```python
from build123d import *

# Parameters (mm, degrees)
SKETCH1_R               = 12
BOSS_EXTRUDE1_DEPTH     = 12
SKETCH9_R               = 14.1
CUT_EXTRUDE2_DEPTH      = 9
SKETCH7_R               = 14
SKETCH7_R_2             = 12
BOSS_EXTRUDE3_DEPTH     = 3
CUT_EXTRUDE5_DEPTH      = 49.191389272
CUT_EXTRUDE5_DEPTH_BACK = 49.191389272
SKETCH12_R              = 1.6
SKETCH13_W              = 2.5
SKETCH13_H              = 1
CUT_EXTRUDE6_DEPTH      = 9
CHAMFER1_SIZE           = 0.6
CHAMFER1_SIZE_2         = 0.661222502


with BuildPart() as part:
    # Sketch1 → Boss-Extrude1 (new body)
    with BuildSketch(Plane.XY):
        with BuildLine():
            Line((-15.1, -38), (-10.1, -38))
            Line((-10.1, -38), (-10.1, -20))
            Line((-10.1, -20), (10.1, -20))
            Line((10.1, -20), (10.1, -38))
            Line((10.1, -38), (15.1, -38))
            Line((15.1, -38), (15.1, -11.029534738))
            ThreePointArc((15.1, -11.029534738), (15.331712472, -8.319532432), (16.020123134, -5.688203124))
            ThreePointArc((16.020123134, -5.688203124), (0, 17), (-16.020123134, -5.688203124))
            ThreePointArc((-16.020123134, -5.688203124), (-15.331712472, -8.319532432), (-15.1, -11.029534738))
            Line((-15.1, -11.029534738), (-15.1, -38))
        make_face()
        Circle(SKETCH1_R, mode=Mode.SUBTRACT)
    extrude(amount=BOSS_EXTRUDE1_DEPTH)

    # Sketch9 → Cut-Extrude2 (cut)
    with BuildSketch(Plane.XY.offset(12)):
        Circle(SKETCH9_R)
    extrude(amount=-CUT_EXTRUDE2_DEPTH, mode=Mode.SUBTRACT)

    # Sketch7 → Boss-Extrude3 (add)
    with BuildSketch(Plane.XY):
        Circle(SKETCH7_R)
        with Locations(Location((0, 0, 0), (0, 0, 180))):
            Circle(SKETCH7_R_2, mode=Mode.SUBTRACT)
    extrude(amount=BOSS_EXTRUDE3_DEPTH)

    # Sketch12 → Cut-Extrude5 (cut, two sides: drawn at the far end of the back side and taken through both)
    with BuildSketch(Plane.ZY.offset(-10.1).offset(-CUT_EXTRUDE5_DEPTH_BACK)):
        with Locations(Location((6, -30, 0), (0, 0, 270))):
            Circle(SKETCH12_R)
    extrude(amount=CUT_EXTRUDE5_DEPTH + CUT_EXTRUDE5_DEPTH_BACK, mode=Mode.SUBTRACT)

    # Sketch13 → Cut-Extrude6 (cut)
    with BuildSketch(Plane.XY.offset(12)):
        with Locations((0, -14.544482903)):
            Rectangle(SKETCH13_W, SKETCH13_H)
    extrude(amount=-CUT_EXTRUDE6_DEPTH, mode=Mode.SUBTRACT)

    # Chamfer1
    # the kernel refuses this chamfer: 0.661222502, 0.6 mm, written as the material it takes off along each edge
    with BuildSketch(Plane(origin=(10.1, -20, 0), x_dir=(0, 0, 1), z_dir=(0, -1, 0)), Plane(origin=(-10.1, -39.543009793, 0), x_dir=(0, 0, 1), z_dir=(0, 1, 0))) as chamfer1_piece_1:
        Polygon((CHAMFER1_SIZE, 0), (0, -CHAMFER1_SIZE), (0, 0), align=None)
    extrude(amount=19.543009793, mode=Mode.SUBTRACT)
    with BuildSketch(Plane(origin=(-10.1, -20, 0), x_dir=(0, 0, 1), z_dir=(1, 0, 0))) as chamfer1_piece_2:
        Polygon((CHAMFER1_SIZE, 0), (0, -CHAMFER1_SIZE), (0, 0), align=None)
    extrude(amount=20.2, mode=Mode.SUBTRACT)
    with BuildSketch(Plane(origin=(-10.1, -39.543009793, 12), x_dir=(0, 0, -1), z_dir=(0, 1, 0)), Plane(origin=(10.1, -20, 12), x_dir=(0, 0, -1), z_dir=(0, -1, 0))) as chamfer1_piece_3:
        Polygon((CHAMFER1_SIZE, 0), (0, CHAMFER1_SIZE), (0, 0), align=None)
    extrude(amount=19.543009793, mode=Mode.SUBTRACT)
    with BuildSketch(Plane(origin=(10.1, -38, -1.543009793), x_dir=(0, 1, 0), z_dir=(0, 0, 1))) as chamfer1_piece_4:
        Polygon((CHAMFER1_SIZE, 0), (0, -CHAMFER1_SIZE), (0, 0), align=None)
    extrude(amount=15.086019586, mode=Mode.SUBTRACT)
    with BuildSketch(Plane(origin=(-10.1, -38, -1.543009793), x_dir=(0, 1, 0), z_dir=(0, 0, 1))) as chamfer1_piece_5:
        Polygon((CHAMFER1_SIZE, 0), (0, CHAMFER1_SIZE), (0, 0), align=None)
    extrude(amount=15.086019586, mode=Mode.SUBTRACT)
    with BuildSketch(Plane(origin=(-10.1, -20, 12), x_dir=(0, 0, -1), z_dir=(1, 0, 0))) as chamfer1_piece_6:
        Polygon((CHAMFER1_SIZE, 0), (0, CHAMFER1_SIZE), (0, 0), align=None)
    extrude(amount=20.2, mode=Mode.SUBTRACT)
    with BuildSketch(Plane(origin=(-1.25, -14.044482903, 13.704300801), x_dir=(0, -1, 0), z_dir=(0, 0, -1))) as chamfer1_piece_7:
        with BuildLine():
            Line((CHAMFER1_SIZE_2, 0), (-0.06766867, 0.609748345))
            ThreePointArc((-0.06766867, 0.609748345), (-0.031575454, 0.314744335), (0, 0))
            Line((0, 0), (CHAMFER1_SIZE_2, 0))
        make_face()
    extrude(amount=10.704300801, mode=Mode.SUBTRACT)
    with BuildSketch(Plane(origin=(1.25, -14.044482903, 13.754921918), x_dir=(0, -1, 0), z_dir=(0, 0, -1))) as chamfer1_piece_8:
        with BuildLine():
            Line((CHAMFER1_SIZE, 0), (-0.07674701, -0.67674701))
            ThreePointArc((-0.07674701, -0.67674701), (-0.035457258, -0.349124916), (0, 0))
            Line((0, 0), (CHAMFER1_SIZE, 0))
        make_face()
    extrude(amount=10.754921918, mode=Mode.SUBTRACT)
    with BuildSketch(Plane(origin=(-10.1, -20, 0), x_dir=(0, 0, 1), z_dir=(1, 0, 0))) as chamfer1_piece_9a_section:
        Polygon((CHAMFER1_SIZE, 0), (0, -CHAMFER1_SIZE), (0, 0), align=None)
    chamfer1_piece_9a = extrude(amount=21.743009793, mode=Mode.PRIVATE)
    chamfer1_piece_9a = split(chamfer1_piece_9a, bisect_by=Plane(origin=(10.1, -20, 0), z_dir=(1, 0, 0)), keep=Keep.TOP, mode=Mode.PRIVATE)
    with BuildSketch(Plane(origin=(10.1, -18.456990207, 0), x_dir=(0, 0, 1), z_dir=(0, -1, 0))) as chamfer1_piece_9b_section:
        Polygon((CHAMFER1_SIZE, 0), (0, -CHAMFER1_SIZE), (0, 0), align=None)
    chamfer1_piece_9b = extrude(amount=19.543009793, mode=Mode.PRIVATE)
    chamfer1_piece_9b = split(chamfer1_piece_9b, bisect_by=Plane(origin=(10.1, -20, 0), z_dir=(0, 1, 0)), keep=Keep.TOP, mode=Mode.PRIVATE)
    chamfer1_piece_9 = chamfer1_piece_9a & chamfer1_piece_9b
    add(chamfer1_piece_9, mode=Mode.SUBTRACT)
    with BuildSketch(Plane(origin=(-10.1, -38, 0), x_dir=(0, 0, 1), z_dir=(0, 1, 0))) as chamfer1_piece_10a_section:
        Polygon((CHAMFER1_SIZE, 0), (0, -CHAMFER1_SIZE), (0, 0), align=None)
    chamfer1_piece_10a = extrude(amount=19.543009793, mode=Mode.PRIVATE)
    chamfer1_piece_10a = split(chamfer1_piece_10a, bisect_by=Plane(origin=(-10.1, -20, 0), z_dir=(0, 1, 0)), keep=Keep.TOP, mode=Mode.PRIVATE)
    with BuildSketch(Plane(origin=(-11.643009793, -20, 0), x_dir=(0, 0, 1), z_dir=(1, 0, 0))) as chamfer1_piece_10b_section:
        Polygon((CHAMFER1_SIZE, 0), (0, -CHAMFER1_SIZE), (0, 0), align=None)
    chamfer1_piece_10b = extrude(amount=21.743009793, mode=Mode.PRIVATE)
    chamfer1_piece_10b = split(chamfer1_piece_10b, bisect_by=Plane(origin=(-10.1, -20, 0), z_dir=(-1, 0, 0)), keep=Keep.TOP, mode=Mode.PRIVATE)
    chamfer1_piece_10 = chamfer1_piece_10a & chamfer1_piece_10b
    add(chamfer1_piece_10, mode=Mode.SUBTRACT)
    with BuildSketch(Plane(origin=(-10.1, -38, 12), x_dir=(0, 0, -1), z_dir=(0, 1, 0))) as chamfer1_piece_11a_section:
        Polygon((CHAMFER1_SIZE, 0), (0, CHAMFER1_SIZE), (0, 0), align=None)
    chamfer1_piece_11a = extrude(amount=19.543009793, mode=Mode.PRIVATE)
    chamfer1_piece_11a = split(chamfer1_piece_11a, bisect_by=Plane(origin=(-10.1, -20, 12), z_dir=(0, 1, 0)), keep=Keep.TOP, mode=Mode.PRIVATE)
    with BuildSketch(Plane(origin=(-11.643009793, -20, 12), x_dir=(0, 0, -1), z_dir=(1, 0, 0))) as chamfer1_piece_11b_section:
        Polygon((CHAMFER1_SIZE, 0), (0, CHAMFER1_SIZE), (0, 0), align=None)
    chamfer1_piece_11b = extrude(amount=21.743009793, mode=Mode.PRIVATE)
    chamfer1_piece_11b = split(chamfer1_piece_11b, bisect_by=Plane(origin=(-10.1, -20, 12), z_dir=(-1, 0, 0)), keep=Keep.TOP, mode=Mode.PRIVATE)
    chamfer1_piece_11 = chamfer1_piece_11a & chamfer1_piece_11b
    add(chamfer1_piece_11, mode=Mode.SUBTRACT)
    with BuildSketch(Plane(origin=(-10.1, -20, 12), x_dir=(0, 0, -1), z_dir=(1, 0, 0))) as chamfer1_piece_12a_section:
        Polygon((CHAMFER1_SIZE, 0), (0, CHAMFER1_SIZE), (0, 0), align=None)
    chamfer1_piece_12a = extrude(amount=21.743009793, mode=Mode.PRIVATE)
    chamfer1_piece_12a = split(chamfer1_piece_12a, bisect_by=Plane(origin=(10.1, -20, 12), z_dir=(1, 0, 0)), keep=Keep.TOP, mode=Mode.PRIVATE)
    with BuildSketch(Plane(origin=(10.1, -18.456990207, 12), x_dir=(0, 0, -1), z_dir=(0, -1, 0))) as chamfer1_piece_12b_section:
        Polygon((CHAMFER1_SIZE, 0), (0, CHAMFER1_SIZE), (0, 0), align=None)
    chamfer1_piece_12b = extrude(amount=19.543009793, mode=Mode.PRIVATE)
    chamfer1_piece_12b = split(chamfer1_piece_12b, bisect_by=Plane(origin=(10.1, -20, 12), z_dir=(0, 1, 0)), keep=Keep.TOP, mode=Mode.PRIVATE)
    chamfer1_piece_12 = chamfer1_piece_12a & chamfer1_piece_12b
    add(chamfer1_piece_12, mode=Mode.SUBTRACT)
    # the kernel refuses this chamfer: 0.661222502, 0.6 mm, written as the material it takes off along each edge
    with BuildSketch(Plane(origin=(0, 0, 12), x_dir=(-0.02220052669057942, -0.9997535379355558, 0), z_dir=(0.9997535379355558, -0.02220052669057942, 0))) as chamfer1_2_piece_1:
        Polygon((14.1 + CHAMFER1_SIZE, 0), (14.1, CHAMFER1_SIZE), (14.1, 0), align=None)
    revolve(axis=Axis((0, 0, 12), (0, 0, -1)), revolution_arc=357.181058693, mode=Mode.SUBTRACT)


solid = part.part
```
Geometry: final body of the model. Coordinates: model frame, mm. A direction names the side the tool comes from. Coordinates: 2 decimals unless noted, no trailing zeros. Order: outer loops, then holes, each group sorted by start corner. A loop starts at its lowest first (then second) coordinate and runs counter-clockwise, first axis right, second up. Notation, with made-up numbers: (-28.75, 50.5) -> (29.25, 50.5) arc R36 cw to (29.25, 85.5) -> close; hole circle Ø3 at (-0.75, -2). An arc over 180 degrees is marked (long way). Answer in a Markdown table with one row per item.
Item 1: Section B-B on y = -23.5. Output: boundary loops of the cut face in (x, z).
Return value:
| item | result |
|---|---|
| outline | (-15.1, 0) -> (-10.7, 0) -> (-10.1, 0.6) -> (-10.1, 11.4) -> (-10.7, 12) -> (-15.1, 12) -> close; (10.1, 0.6) -> (10.7, 0) -> (15.1, 0) -> (15.1, 12) -> (10.7, 12) -> (10.1, 11.4) -> close |
Item 2: Contact query for flat-ended pins moving along their axis: P1, Ø3, axis at y = -25, z = 4.5, coming from the -X side; P2, Ø4, axis at y = -30, z = 6, coming from the +X side; P3, Ø1.5, axis at y = 4.5, z = 5.5, coming from the -X side; P4, Ø3, axis at x = -12, y = 2.5, coming from the -Z side. Output: stop coordinate, or through.
Return value:
| item | result |
|---|---|
| P1 | stops at x = -15.1 |
| P2 | stops at x = 15.1 |
| P3 | stops at x = -16.58 |
| P4 | stops at z = 0 |
Item 3: Ray query, L1, parallel to Z at x = 12.75, y = -30; L2, parallel to X at y = -34.5, z = 4.25; L3, parallel to X at y = 0, z = 1.75. Return the intervals inside material, ascending.
Return value:
| item | result |
|---|---|
| L1 | z = 0 to 4.4, 7.6 to 12 |
| L2 | x = -15.1 to -10.1, 10.1 to 15.1 |
| L3 | x = -17 to -12, 12 to 17 |
Item 4: Section C-C on z = 6. Output: boundary loops of the cut face in (x, y).
Return value:
| item | result |
|---|---|
| outline | (-16.02, -5.69) arc R15.96 cw to (-15.1, -11.03) -> (-15.1, -28.4) -> (-10.1, -28.4) -> (-10.1, -20) -> (10.1, -20) -> (10.1, -28.4) -> (15.1, -28.4) -> (15.1, -11.03) arc R15.96 cw to (16.02, -5.69) arc R17 ccw (long way) to start; (-15.1, -38) -> (-10.7, -38) -> (-10.1, -37.4) -> (-10.1, -31.6) -> (-15.1, -31.6) -> close; (10.1, -37.4) -> (10.7, -38) -> (15.1, -38) -> (15.1, -31.6) -> (10.1, -31.6) -> close; hole (-1.86, -13.98) -> (-1.25, -14.71) -> (-1.25, -15.04) -> (1.25, -15.04) -> (1.25, -14.64) -> (1.93, -13.97) arc R14.1 ccw (long way) to start |
Item 5: Access query for faces 4 (the flat face through (15.1, -25, 6)), 5 (the flat face through (3.7, -14.4, 12)), 6 (the flat face through (0, -20, 6)), 7 (the flat face through (0, -15.044, 8)), 8 (the flat face through (-15.1, -24, 6)). Directions: +Z, -Z, +X, -X, +Y, -Y. A direction counts if a zero-diameter tool reaches every point of the face in a straight line with its end or side. Return the directions, or none.
Return value:
| item | result |
|---|---|
| face 4 | +Z, -Z, +X, -Y |
| face 5 | +Z, +X, -X, +Y, -Y |
| face 6 | +Z, -Z, -Y |
| face 7 | +Z |
| face 8 | +Z, -Z, -X, -Y |
Item 6: Section D-D on y = -30. Output: boundary loops of the cut face in (x, z).
Return value:
| item | result |
|---|---|
| outline | (-15.1, 0) -> (-10.7, 0) -> (-10.1, 0.6) -> (-10.1, 4.4) -> (-15.1, 4.4) -> close; (-15.1, 7.6) -> (-10.1, 7.6) -> (-10.1, 11.4) -> (-10.7, 12) -> (-15.1, 12) -> close; (10.1, 0.6) -> (10.7, 0) -> (15.1, 0) -> (15.1, 4.4) -> (10.1, 4.4) -> close; (10.1, 7.6) -> (15.1, 7.6) -> (15.1, 12) -> (10.7, 12) -> (10.1, 11.4) -> close |
Item 7: Draft query along Y for faces 1 (the cylindrical face through (0, 17, 6)), 2 (the cylindrical face through (0.56, 14.09, 7.26)), 3 (the flat face through (-13, -38, 6)). Return one class per face: released by +Y, released by -Y, zero draft, split by the parting line, or undercut.
Return value:
| item | result |
|---|---|
| face 1 | split by the parting line |
| face 2 | undercut |
| face 3 | released by -Y |
Item 8: Section A-A on x = 0. Output: boundary loops of the cut face in (y, z).
Return value:
| item | result |
|---|---|
| outline | (-20, 0.6) -> (-19.4, 0) -> (-12, 0) -> (-12, 3) -> (-15.04, 3) -> (-15.04, 12) -> (-19.4, 12) -> (-20, 11.4) -> close; (12, 0) -> (17, 0) -> (17, 12) -> (14.7, 12) -> (14.1, 11.4) -> (14.1, 3) -> (12, 3) -> close |
